```python
from build123d import *

# Parameters (mm, degrees)
SKETCH1_W           = 42
SKETCH1_H           = 42
BOSS_EXTRUDE1_DEPTH = 16
CUT_EXTRUDE1_DEPTH  = 13
SKETCH3_R           = 3.6
SKETCH3_R_2         = 1.6
CUT_EXTRUDE2_DEPTH  = 62.514225997
SKETCH4_W           = 11
SKETCH4_H           = 7
SKETCH4_W_2         = 7
CUT_EXTRUDE3_DEPTH  = 61.802960454
FILLET2_R           = 1
FILLET3_R           = 4
FILLET4_R           = 4
FILLET5_R           = 4
FILLET6_R           = 1
FILLET7_R           = 1
FILLET8_R           = 1
FILLET10_R          = 1
FILLET11_R          = 1
FILLET12_R          = 1
FILLET13_R          = 1
FILLET14_R          = 1
FILLET15_R          = 1
FILLET16_R          = 1
FILLET17_R          = 1
FILLET18_R          = 1
FILLET19_R          = 2
FILLET20_R          = 2
FILLET21_R          = 2
FILLET22_R          = 2


with BuildPart() as part:
    # Sketch1 → Boss-Extrude1 (new body)
    with BuildSketch(Plane.XY):
        with Locations((21, 21)):
            Rectangle(SKETCH1_W, SKETCH1_H)
    extrude(amount=BOSS_EXTRUDE1_DEPTH)

    # Sketch2 → Cut-Extrude1 (cut)
    with BuildSketch(Plane.XY.offset(16)):
        Polygon((3, 42), (3, 39), (0, 39), (0, 36), (6, 36), (6, 42), align=None)
        Polygon((9, 42), (9, 33), (0, 33), (0, 30), (12, 30), (12, 42), align=None)
        Polygon((15, 42), (15, 27), (0, 27), (0, 24), (18, 24), (18, 42), align=None)
        Polygon((0, 21), (21, 21), (21, 42), (24, 42), (24, 18), (0, 18), align=None)
        Polygon((28, 42), (28, 14), (0, 14), (0, 11), (31, 11), (31, 42), align=None)
        Polygon((35, 42), (35, 7), (0, 7), (0, 4), (38, 4), (38, 42), align=None)
    extrude(amount=-CUT_EXTRUDE1_DEPTH, mode=Mode.SUBTRACT)

    # Sketch3 → Cut-Extrude2 (cut, through all)
    with BuildSketch(Plane(origin=(0, 0, 0), x_dir=(-1, 0, 0), z_dir=(0, 0, -1))):
        with Locations((-21, 21)):
            Circle(SKETCH3_R)
        with Locations((-5.5, 5.5)):
            Circle(SKETCH3_R_2)
        with Locations((-36.5, 5.5)):
            Circle(SKETCH3_R_2)
    extrude(amount=-CUT_EXTRUDE2_DEPTH, mode=Mode.SUBTRACT)

    # Sketch4 → Cut-Extrude3 (cut, through all)
    with BuildSketch(Plane.XY.offset(3)):
        with Locations((5.5, 5.5)):
            Rectangle(SKETCH4_W, SKETCH4_H)
        with Locations((36.5, 5.5)):
            Rectangle(SKETCH4_W_2, SKETCH4_H)
    extrude(amount=CUT_EXTRUDE3_DEPTH, mode=Mode.SUBTRACT)

    # Fillet2
    fillet2_edges = [part.edges().sort_by_distance(p)[0] for p in [
        (3, 39, 9.5),
    ]]
    fillet(fillet2_edges, radius=FILLET2_R)

    # Fillet3
    fillet3_edges = [part.edges().sort_by_distance(p)[0] for p in [
        (9, 33, 9.5),
    ]]
    fillet(fillet3_edges, radius=FILLET3_R)

    # Fillet4
    fillet4_edges = [part.edges().sort_by_distance(p)[0] for p in [
        (15, 27, 9.5),
    ]]
    fillet(fillet4_edges, radius=FILLET4_R)

    # Fillet5
    fillet5_edges = [part.edges().sort_by_distance(p)[0] for p in [
        (28, 14, 9.5),
    ]]
    fillet(fillet5_edges, radius=FILLET5_R)

    # Fillet6
    fillet6_edges = [part.edges().sort_by_distance(p)[0] for p in [
        (35, 9, 9.5),
    ]]
    fillet(fillet6_edges, radius=FILLET6_R)

    # Fillet7
    fillet7_edges = [part.edges().sort_by_distance(p)[0] for p in [
        (33, 7, 9.5),
    ]]
    fillet(fillet7_edges, radius=FILLET7_R)

    # Fillet8
    fillet8_edges = [part.edges().sort_by_distance(p)[0] for p in [
        (40, 2, 9.5),
    ]]
    fillet(fillet8_edges, radius=FILLET8_R)

    # Fillet10
    fillet10_edges = [part.edges().sort_by_distance(p)[0] for p in [
        (33, 9, 9.5),
    ]]
    fillet(fillet10_edges, radius=FILLET10_R - 0.0001)  # a hair under: the kernel refuses the full size

    # Fillet11
    fillet11_edges = [part.edges().sort_by_distance(p)[0] for p in [
        (38, 9, 9.5),
    ]]
    fillet(fillet11_edges, radius=FILLET11_R)

    # Fillet12
    fillet12_edges = [part.edges().sort_by_distance(p)[0] for p in [
        (40, 9, 9.5),
    ]]
    fillet(fillet12_edges, radius=FILLET12_R - 0.0001)  # a hair under: the kernel refuses the full size

    # Fillet13
    fillet13_edges = [part.edges().sort_by_distance(p)[0] for p in [
        (33, 2, 9.5),
    ]]
    fillet(fillet13_edges, radius=FILLET13_R)

    # Fillet14
    fillet14_edges = [part.edges().sort_by_distance(p)[0] for p in [
        (33, 4, 9.5),
    ]]
    fillet(fillet14_edges, radius=FILLET14_R - 0.0001)  # a hair under: the kernel refuses the full size

    # Fillet15
    fillet15_edges = [part.edges().sort_by_distance(p)[0] for p in [
        (11, 4, 9.5),
    ]]
    fillet(fillet15_edges, radius=FILLET15_R)

    # Fillet16
    fillet16_edges = [part.edges().sort_by_distance(p)[0] for p in [
        (11, 2, 9.5),
    ]]
    fillet(fillet16_edges, radius=FILLET16_R - 0.0001)  # a hair under: the kernel refuses the full size

    # Fillet17
    fillet17_edges = [part.edges().sort_by_distance(p)[0] for p in [
        (11, 7, 9.5),
    ]]
    fillet(fillet17_edges, radius=FILLET17_R)

    # Fillet18
    fillet18_edges = [part.edges().sort_by_distance(p)[0] for p in [
        (11, 9, 9.5),
    ]]
    fillet(fillet18_edges, radius=FILLET18_R - 0.0001)  # a hair under: the kernel refuses the full size

    # Fillet19
    fillet19_edges = [part.edges().sort_by_distance(p)[0] for p in [
        (6, 36, 9.5),
    ]]
    fillet(fillet19_edges, radius=FILLET19_R)

    # Fillet20
    fillet20_edges = [part.edges().sort_by_distance(p)[0] for p in [
        (12, 30, 9.5),
    ]]
    fillet(fillet20_edges, radius=FILLET20_R)

    # Fillet21
    fillet21_edges = [part.edges().sort_by_distance(p)[0] for p in [
        (18, 24, 9.5),
    ]]
    fillet(fillet21_edges, radius=FILLET21_R)

    # Fillet22
    fillet22_edges = [part.edges().sort_by_distance(p)[0] for p in [
        (31, 11, 9.5),
    ]]
    fillet(fillet22_edges, radius=FILLET22_R)


solid = part.part
```
Here's how the part is built. I have some questions about the finished solid (model axes, mm). A direction names the side the tool comes from. Round coordinates to 2 decimals unless told otherwise and drop trailing zeros. Order: outer loops, then holes, each group sorted by start corner. A loop starts at its lowest first (then second) coordinate and runs counter-clockwise, first axis right, second up. Notation, with made-up numbers: M 4.25,76 L 61.25,76 A13 cw 61.25,100 Z; hole C -30,84 d7. An arc over 180 degrees is marked long. Use CSV: the item, a comma, the result in double quotes.
1) I want a section at B-B (y = 5.5). List the corners of the cut face in (x, z) for me.
Taken from the geometry:
outline,"M 0,0 L 3.9,0 L 3.9,3 L 0,3 Z; M 7.1,0 L 34.9,0 L 34.9,3 L 7.1,3 Z; M 38.1,0 L 42,0 L 42,16 L 40,16 L 40,3 L 38.1,3 Z"
2) I want a section at C-C (z = 2). List the corners of the cut face in (x, y) for me, then the cut area to 3 significant figures.
Taken from the geometry:
outline,"M 0,0 L 42,0 L 42,42 L 0,42 Z; hole C 5.5,5.5 d3.2; hole C 21,21 d7.2; hole C 36.5,5.5 d3.2"
area,"1,710 mm^2"
3) I need wall thicknesses on line 1 along X through (y, z) = (3, 15.25); line 2 along Y through (x, z) = (12.5, 13.5); line 3 along X through (y, z) = (17, 3.5). Which ranges of each line are inside material? Lowest first, please. Write a range as [from, to].
Taken from the geometry:
line 1,"[11, 33], [40, 42]"
line 2,"[0, 4], [7, 11], [14, 18], [21, 24], [27.29, 42]"
line 3,"[0, 27.87], [31, 35], [38, 42]"
4) I want a section at D-D (x = 15.5). List the corners of the cut face in (y, z) for me.
Taken from the geometry:
outline,"M 0,0 L 42,0 L 42,3 L 24,3 L 24,16 L 21,16 L 21,3 L 18,3 L 18,16 L 14,16 L 14,3 L 11,3 L 11,16 L 7,16 L 7,3 L 4,3 L 4,16 L 0,16 Z"
5) I want a section at A-A (x = 36.5). List the corners of the cut face in (y, z) for me, then the cut area to 3 significant figures.
Taken from the geometry:
outline,"M 0,0 L 3.9,0 L 3.9,3 L 2,3 L 2,16 L 0,16 Z; M 7.1,0 L 42,0 L 42,3 L 7.1,3 Z"
area,"142 mm^2"
6) On a 3-axis mill with a long thin cutter (end or side, diameter ignored), from which of +Z, -Z, +X, -X, +Y, -Y can I reach the whole of each face in a straight line? I mean faces 4 (the flat face through (13.6, 23.8, 16)), 5 (the cylindrical face through (11.43, 30.6, 9.41)), 6 (the flat face through (12, 14, 10)), 7 (the flat face through (3, 41, 10)), 8 (the flat face through (40, 5, 9)). Say none if no direction works.
Taken from the geometry:
face 4,"+Z, +X, -X, +Y, -Y"
face 5,"+Z, -X, +Y"
face 6,"+Z, -X"
face 7,"+Z, +Y"
face 8,"+Z"
7) If we mould it in two halves opening along Y, with no side actions, what happens to faces 1 (the flat face through (23.5, 18, 9.6)), 2 (the cylindrical face through (11.285, 7.301, 9.591)), 3 (the flat face through (6, 40, 10))? For each: pulls with the +Y half, pulls with the -Y half, needs draft (parallel to the pull), parting line crosses it, or undercut.
Taken from the geometry:
face 1,"pulls with the +Y half"
face 2,"undercut"
face 3,"needs draft"
